Here's the drawing with two shaded views (mm, measured from the low corner). I have some questions. Coordinates: 2 decimals unless noted, no trailing zeros. Write each loop counter-clockwise with the first axis right and the second up, starting at its lowest first coordinate (ties: lowest second). Pieces come first, ordered by that corner, then holes.
Item 1: I want a section at C-C on x = 3.9. Please give me the cut outline in (y, z).
Item 2: For P1, Ø1.5, axis at x = 4, y = 1, coming from the -Z side, with a flat end and sliding along its axis, tell me the tip position at first contact or that it passes through.
Item 3: I want a section at D-D on x = 2. Please give me the cut outline in (y, z).
Item 4: Thinking about a two-plate mould opening in Y: for the marked faces 1, 2 and 3, which applies, +Y half, -Y half, draft (parallel to the pull), parting line (faces both ways), or undercut?
Item 5: If I drill on probe 1 along X at (y, z) = (4.5, 0.6); probe 2 along Y at (x, z) = (3.9, 0.3); probe 3 along X at (y, z) = (3.5, 0.65) (3 decimals), over which ranges is the centre line in solid material (lowest first)?
Item 6: I want a section at A-A on y = 3.9. Please give me the cut outline in (x, z) (3 decimals), then the cut area to 3 significant figures.
Item 7: I want a section at B-B on z = 0.2. Please give me the cut outline in (x, y) (3 decimals).
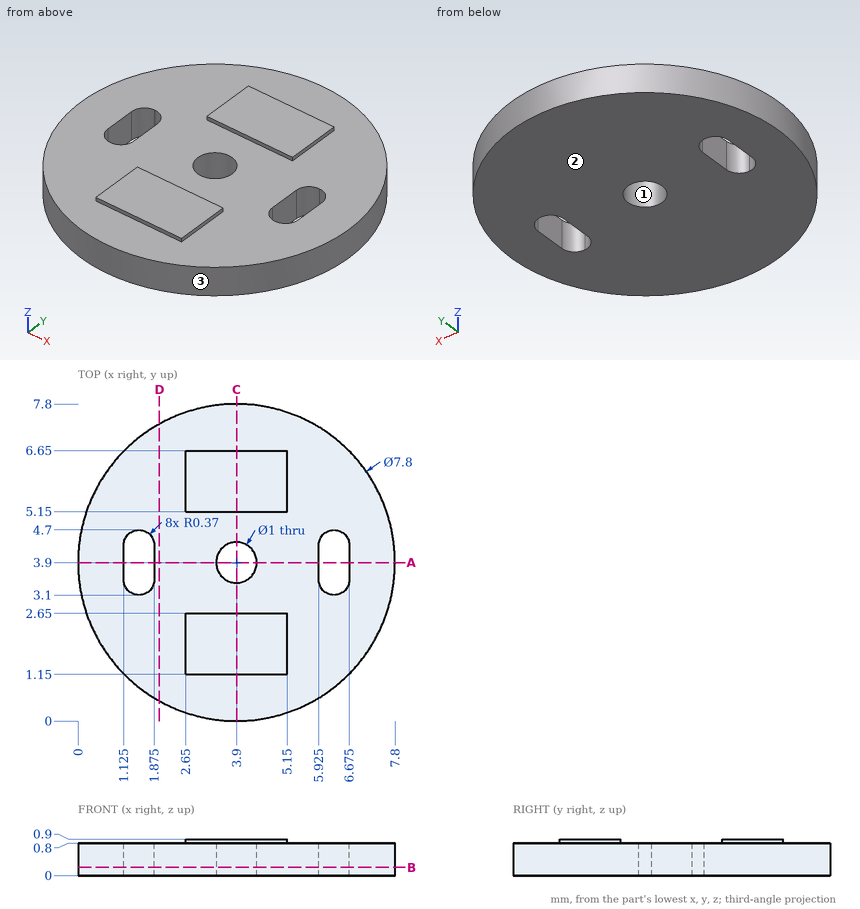
Response values:
1. outline: (0, 0) - (3.4, 0) - (3.4, 0.8) - (2.65, 0.8) - (2.65, 0.9) - (1.15, 0.9) - (1.15, 0.8) - (0, 0.8) - close; (4.4, 0) - (7.8, 0) - (7.8, 0.8) - (6.65, 0.8) - (6.65, 0.9) - (5.15, 0.9) - (5.15, 0.8) - (4.4, 0.8) - close
2. P1: stops at z = 0
3. outline: (0.49, 0) - (7.31, 0) - (7.31, 0.8) - (0.49, 0.8) - close
4. face 1: undercut
4. face 2: draft
4. face 3: parting line
5. probe 1: x = 0.05 to 1.17, 1.83 to 5.97, 6.63 to 7.75
5. probe 2: y = 0 to 3.4, 4.4 to 7.8
5. probe 3: x = 0.021 to 1.125, 1.875 to 3.6, 4.2 to 5.925, 6.675 to 7.779
6. outline: (0, 0) - (1.125, 0) - (1.125, 0.8) - (0, 0.8) - close; (1.875, 0) - (3.4, 0) - (3.4, 0.8) - (1.875, 0.8) - close; (4.4, 0) - (5.925, 0) - (5.925, 0.8) - (4.4, 0.8) - close; (6.675, 0) - (7.8, 0) - (7.8, 0.8) - (6.675, 0.8) - close
6. area: 4.24 mm2
7. outline: circle Ø7.8 at (3.9, 3.9); hole (1.125, 3.47) arc R0.37 ccw to (1.495, 3.1) - (1.505, 3.1) arc R0.37 ccw to (1.875, 3.47) - (1.875, 4.33) arc R0.37 ccw to (1.505, 4.7) - (1.495, 4.7) arc R0.37 ccw to (1.125, 4.33) - close; hole circle Ø1 at (3.9, 3.9); hole (5.925, 3.47) arc R0.37 ccw to (6.295, 3.1) - (6.305, 3.1) arc R0.37 ccw to (6.675, 3.47) - (6.675, 4.33) arc R0.37 ccw to (6.305, 4.7) - (6.295, 4.7) arc R0.37 ccw to (5.925, 4.33) - close
